The listing builds one solid part. Answer for the finished solid, in the listing's coordinates (mm). Face numbers are marked on the shaded views. Coordinates: 2 decimals unless noted, no trailing zeros. Write each loop counter-clockwise with the first axis right and the second up, starting at its lowest first coordinate (ties: lowest second). Pieces come first, ordered by that corner, then holes.
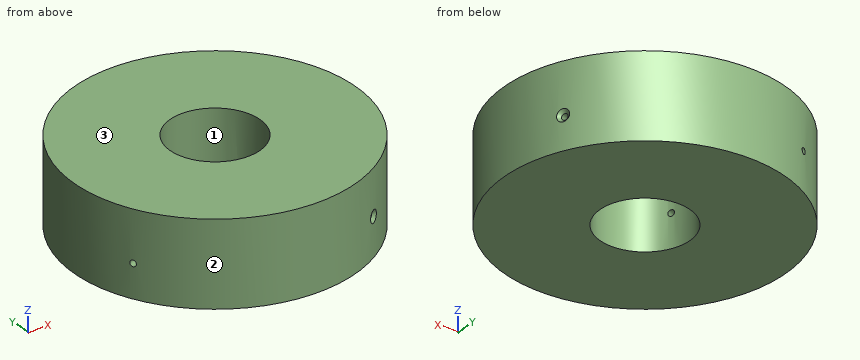
from build123d import *

# Parameters (mm, degrees)
SKETCH2_R                                           = 50
SKETCH2_R_2                                         = 16
BOSS_EXTRUDE1_DEPTH                                 = 30
CSK_FOR_M2_COUNTERSUNK_FLAT_HEAD_SCREW1_D           = 2.2
CSK_FOR_M2_COUNTERSUNK_FLAT_HEAD_SCREW1_CSINK_D     = 4.4
CSK_FOR_M2_COUNTERSUNK_FLAT_HEAD_SCREW1_CSINK_ANGLE = 90
CSK_FOR_M2_COUNTERSUNK_FLAT_HEAD_SCR_2_D            = 2.2
CSK_FOR_M2_COUNTERSUNK_FLAT_HEAD_SCR_2_CSINK_D      = 4.4
CSK_FOR_M2_COUNTERSUNK_FLAT_HEAD_SCR_2_CSINK_ANGLE  = 90


with BuildPart() as part:
    # Sketch2 → Boss-Extrude1 (new body)
    with BuildSketch(Plane.XY):
        Circle(SKETCH2_R)
        Circle(SKETCH2_R_2, mode=Mode.SUBTRACT)
    extrude(amount=BOSS_EXTRUDE1_DEPTH)

    # CSK for M2 Countersunk Flat Head Screw1 (through all)
    with Locations(Plane(origin=(24.873497254, -43.374060617, 13.771522771), x_dir=(-0.86748121233, -0.497469945076, 0), z_dir=(0.497469945076, -0.86748121233, 0))):
        with Locations((0, 0)):
            CounterSinkHole(CSK_FOR_M2_COUNTERSUNK_FLAT_HEAD_SCREW1_D / 2, CSK_FOR_M2_COUNTERSUNK_FLAT_HEAD_SCREW1_CSINK_D / 2, counter_sink_angle=CSK_FOR_M2_COUNTERSUNK_FLAT_HEAD_SCREW1_CSINK_ANGLE)

    # CSK for M2 Countersunk Flat Head Scr 2 (through all)
    with Locations(Plane(origin=(45.576703695, 20.561227598, 11.889158969), x_dir=(-0.411224951932, 0.91153389345, 0), z_dir=(0.91153389345, 0.411224951932, 0))):
        with Locations((0, 0)):
            CounterSinkHole(CSK_FOR_M2_COUNTERSUNK_FLAT_HEAD_SCR_2_D / 2, CSK_FOR_M2_COUNTERSUNK_FLAT_HEAD_SCR_2_CSINK_D / 2, counter_sink_angle=CSK_FOR_M2_COUNTERSUNK_FLAT_HEAD_SCR_2_CSINK_ANGLE)


solid = part.part
Q1. The part is cut by section C-C, the plane z = 22. Write down the section's boundary in (x, y).
Answers below:
outline: circle Ø100 at (0, 0); hole circle Ø32 at (0, 0)
Q2. Determine the mould class of the marked faces 1, 2 and 3 for opening direction Y: released by +Y, released by -Y, zero draft, split by the parting line, or undercut.
Answers below:
face 1: undercut
face 2: split by the parting line
face 3: zero draft
Q3. Find the intervals of material crossed by probe 1 along Y at (x, z) = (0, 23); probe 2 along Z at (x, y) = (14, -25.5); probe 3 along Y at (x, z) = (-1.5, 16), in increasing order.
Answers below:
probe 1: y = -50 to -16, 16 to 50
probe 2: z = 0 to 12.81, 14.73 to 30
probe 3: y = -49.98 to -15.93, 15.93 to 49.98
Q4. Given pin 1 (1 mm diameter, centred on x = 6, z = 4.5, fed in from +Y); pin 2 (6 mm diameter, centred on x = -5.5, z = 21.5, fed in from -Y); pin 3 (8 mm diameter, centred on x = 36.5, z = 24, fed in from +Y), each flat-ended and moving along its own axis, determine where each tip first touches the part or whether it passes through.
Answers below:
pin 1: stops at y = 49.7
pin 2: stops at y = -49.94
pin 3: stops at y = 38
Q5. The part is cut by section A-A, the plane x = 0. Write down the section's boundary in (y, z).
Answers below:
outline: (-50, 0) - (-16, 0) - (-16, 30) - (-50, 30) - close; (16, 0) - (50, 0) - (50, 30) - (16, 30) - close
